Check sheet for the drawn part. Datum: minimum x, y, z corner. Units: mm. Coordinates: 2 decimals unless noted, no trailing zeros. Loops run counter-clockwise (first coordinate to the right, second up) from the corner with the lowest first, then second, coordinate; pieces in that order, holes last.
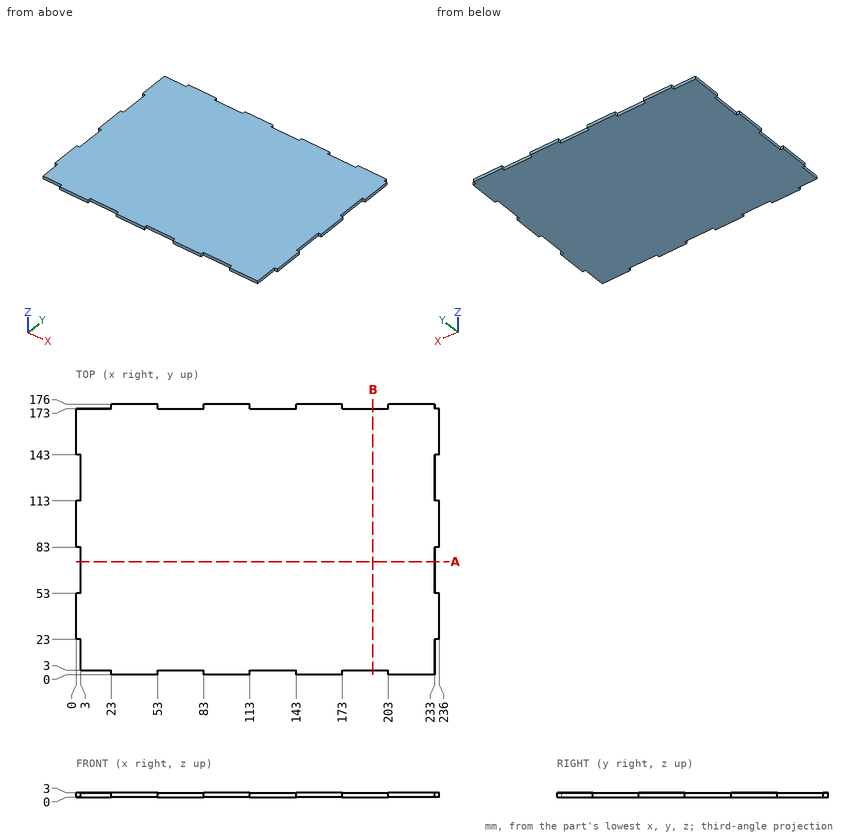
(1) Sectioned sample at B-B on x = 193. Record the cut outline in (y, z).
Findings:
outline: (3, 0) - (173, 0) - (173, 3) - (3, 3) - close
(2) Sectioned sample at A-A on y = 73.5. Record the cut outline in (x, z), and give its area (3 significant figures).
Findings:
outline: (3, 0) - (233, 0) - (233, 3) - (3, 3) - close
area: 690 mm2
(3) Scan lines: L1, parallel to Y at x = 13, z = 1.7; L2, parallel to X at y = 60, z = 1.25. Record each from-to range of solid material in increasing order.
Findings:
L1: y = 3 to 173
L2: x = 3 to 233
(4) Gauge pin test, flat ends, axial feed: pin 1 Ø0.9 at (y, z) = (174, 1.5) entering from +X; pin 2 Ø0.9 at (y, z) = (1.5, 1.5) entering from -X; pin 3 Ø1.5 at (x, z) = (194.5, 2) entering from +Y. Record the tip position at first contact, or that the pin passes through.
Findings:
pin 1: stops at x = 233
pin 2: stops at x = 23
pin 3: stops at y = 173
